The listing builds one solid part. Answer for the finished solid, in the listing's coordinates (mm). Face numbers are marked on the shaded views. Coordinates: 2 decimals unless noted, no trailing zeros. Loops run counter-clockwise (first coordinate to the right, second up) from the corner with the lowest first, then second, coordinate; pieces in that order, holes last. Notation, with made-up numbers: M 61.25,73.5 L 91.25,73.5 A15 ccw 91.25,85.5 Z; hole C -20,10.5 d4. An arc over 180 degrees is marked long. Answer as a JSON object with one key per item and string values. Group by question number.
1. Given pin 1 (8 mm diameter, centred on y = 377, z = 15, fed in from +X); pin 2 (2.5 mm diameter, centred on x = 435, y = 145, fed in from +Z); pin 3 (4.5 mm diameter, centred on x = 417, z = 12.5, fed in from +Y), each flat-ended and moving along its own axis, determine where each tip first touches the part or whether it passes through.
2. Determine the mould class of the marked faces 1 and 2 for opening direction Y: released by +Y, released by -Y, zero draft, split by the parting line, or undercut.
3. A cutting plane is placed at B-B on x = 222. Give the vertices of the cut face in (y, z), and give its area (3 significant figures).
4. A cutting plane is placed at A-A on y = 39. Give the vertices of the cut face in (x, z).
5. Straight lines are drawn through the part: L1, parallel to X at y = 5, z = 15.5; L2, parallel to Y at x = 435, z = 14; L3, parallel to X at y = 145, z = 14.5. For each, find the intervals that lie inside material, in ascending order.
Autodesk Fusion 360 part; units mm, degrees
sketch "Sketch1" plane through (0, 0, 0) normal (0, 0, 1) x (1, 0, 0)
  line L0 (0, 0) -> (390, 0)
  line L1 (390, 0) -> (390, 390)
  line L2 (390, 390) -> (0, 390)
  line L3 (0, 390) -> (0, 0)
  line L4 (390, 0) -> (440, 0)
  line L5 (440, 0) -> (440, 150)
  line L6 (440, 150) -> (390, 150)
  line L7 (390, 150) -> (390, 0)
  dimension "d5" = 390
  dimension "d6" = 390
  dimension "d23" = 150
  dimension "d26" = 50
extrude "Extrude1" add sketch "Sketch1" along normal blind 18
fillet "Fillet2" radius 5 3 edges at (440, 0, 9) (440, 150, 9) (390, 150, 9)
sketch "Sketch4" plane through (0, 0, 18) normal (0, 0, 1) x (-1, 0, 0)
  arc A0 (-440, -145) -> (-435, -150) centre (-435, -145) ccw
  line L0 (-435, -150) -> (-395, -150)
  arc A1 (-390, -155) -> (-395, -150) centre (-395, -155) ccw
  line L1 (-390, -155) -> (-390, -390)
  line L2 (-390, -390) -> (0, -390)
  line L3 (0, -390) -> (0, 0)
  line L4 (0, 0) -> (-435, 0)
  arc A2 (-435, 0) -> (-440, -5) centre (-435, -5) ccw
  line L5 (-440, -5) -> (-440, -145)
  line L6 (-400, -148) -> (-430, -148)
  line L7 (-430, -148) -> (-430, -10)
  line L8 (-430, -10) -> (-400, -10)
  line L9 (-400, -10) -> (-400, -148)
  point P0 (-395, -145)
  point P1 (-435, -145)
  point P2 (-435, -5)
  point P3 (-395, -5)
  dimension "d28" = 10
  dimension "d29" = 10
  dimension "d30" = 10
  dimension "d38" = 2
  dimension "d50" = 5
  dimension "d51" = 5
  dimension "d52" = 5
  dimension "d53" = 5
  dimension "d54" = 5
  dimension "d55" = 45
  dimension "d59" = 45
extrude "Extrude4" cut sketch "Sketch4" against normal blind 14.4 contours L6 L7 L8 L9
fillet "Fillet3" radius 5 4 edges at (400, 10, 10.8) (430, 10, 10.8) (400, 148, 10.8) (430, 148, 10.8)
sketch "Sketch5" plane through (0, 0, 18) normal (0, 0, 1) x (-1, 0, 0)
  line L0 (-400, -15) -> (-400, -143)
  arc A0 (-390, -155) -> (-395, -150) centre (-395, -155) ccw
  line L1 (-390, -155) -> (-390, -390)
  line L2 (-390, -390) -> (0, -390)
  line L3 (0, -390) -> (0, 0)
  line L4 (0, 0) -> (-435, 0)
  arc A1 (-435, 0) -> (-440, -5) centre (-435, -5) ccw
  line L5 (-440, -5) -> (-440, -145)
  arc A2 (-440, -145) -> (-435, -150) centre (-435, -145) ccw
  line L6 (-435, -150) -> (-395, -150)
  line L7 (-430, -143) -> (-430, -15)
  arc A3 (-425, -10) -> (-430, -15) centre (-425, -15) ccw
  line L8 (-425, -10) -> (-405, -10)
  arc A4 (-400, -15) -> (-405, -10) centre (-405, -15) ccw
  line L9 (-24, -366) -> (-366, -366)
  line L10 (-366, -366) -> (-366, -24)
  line L11 (-366, -24) -> (-24, -24)
  line L12 (-24, -24) -> (-24, -366)
  line L13 (-405, -148) -> (-425, -148)
  arc A5 (-405, -148) -> (-400, -143) centre (-405, -143) ccw
  arc A6 (-430, -143) -> (-425, -148) centre (-425, -143) ccw
  line L14 (-316, -366) -> (-316, -390)
  line L15 (-316, -390) -> (-286, -390)
  line L16 (-286, -390) -> (-286, -366)
  line L17 (-366, -120) -> (-400, -120)
  line L18 (-400, -120) -> (-400, -110)
  line L19 (-400, -110) -> (-366, -110)
  line L20 (-366, -110) -> (-366, -120)
  dimension "d34" = 342
  dimension "d35" = 342
  dimension "d36" = 24
  dimension "d37" = 24
  dimension "d41" = 50
  dimension "d42" = 30
  dimension "d60" = 30
  dimension "d61" = 10
extrude "Extrude5" cut sketch "Sketch5" against normal blind 10 contours L0 L10 L17 L18 L19 L20 | L9 L10 L11 L12 L20 | L2 L9 L14 L15 L16
fillet "Fillet4" radius 5 8 edges at (24, 366, 13) (286, 366, 13) (24, 24, 13) (366, 24, 13) (366, 366, 13) (316, 366, 13) (316, 390, 13) (286, 390, 13)
fillet "Fillet4" radius 5 4 edges at (366, 120, 13) (400, 120, 13) (366, 110, 13) (400, 110, 13)
sketch "Sketch6" plane through (0, 150, 0) normal (0, 1, 0) x (-1, 0, 0)
  line L0 (-395, 0) -> (-395, 18)
  line L1 (-435, 18) -> (-435, 0)
  line L2 (-435, 0) -> (-395, 0)
  line L3 (-440, 18) -> (-440, 0)
  line L4 (-395, 18) -> (-435, 18)
  point P0 (-415, 10)
  dimension "d45" = 25
  dimension "d46" = 10
hole "Hole1" at (415, 150, 10) direction (0, -1, 0) diameter 10 depth 2 tip angle 118
hole "Hole2" at (395, 5, 18) at (435, 5, 18) at (435, 145, 18) at (395, 145, 18) direction (0, 0, -1) diameter 3 depth 10 tip angle 118
equation "t_base = 18 mm"
equation "a_ramme = 20 mm"
equation "d5 = d + 2 * a_ramme"
equation "d6 = b + 2 * a_ramme"
equation "d7 = t_base"
equation "a_outlet = 30 mm"
equation "d23 = d_utilites"
equation "b_utilities = 50 mm"
equation "d_utilites = 150 mm"
equation "d26 = b_utilities"
equation "d31 = -t_base * 0.8"
equation "d34 = b - 2 * t"
equation "d35 = d - 2 * t"
equation "d36 = a_ramme + t"
equation "d37 = a_ramme + t"
equation "d42 = a_outlet"
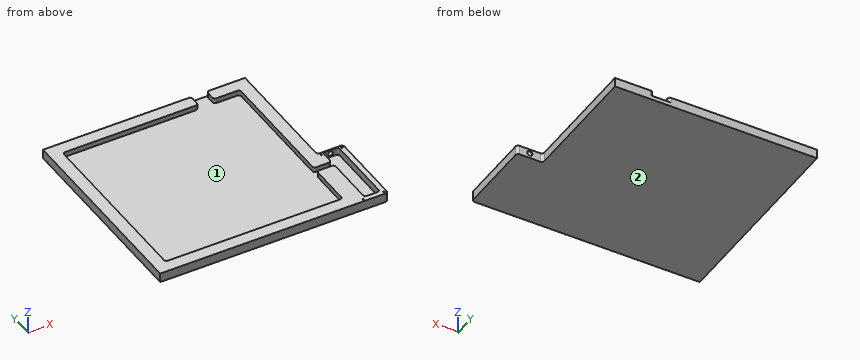
From the geometry:
{
 "1": {"pin 1": "stops at x = 390", "pin 2": "stops at z = 7.85", "pin 3": "stops at y = 150"},
 "2": {"face 1": "undercut", "face 2": "zero draft"},
 "3": {"outline": "M 0,0 L 390,0 L 390,18 L 366,18 L 366,8 L 24,8 L 24,18 L 0,18 Z", "area": "3,600 mm²"},
 "4": {"outline": "M 0,0 L 440,0 L 440,18 L 430,18 L 430,3.6 L 400,3.6 L 400,18 L 366,18 L 366,8 L 24,8 L 24,18 L 0,18 Z"},
 "5": {"L1": "x = 0 to 393.5, 396.5 to 433.5, 436.5 to 440", "L2": "y = 0 to 3.5, 6.5 to 143.5, 146.5 to 150", "L3": "x = 0 to 24, 366 to 393.5, 396.5 to 400.42, 429.58 to 433.5, 436.5 to 440"}
}
